from build123d import *

# Parameters (mm, degrees)
FILLET1_R = 2.54


with BuildPart() as part:
    # Sketch1 → Revolve2 (revolve)
    with BuildSketch(Plane.XY):
        Polygon((0, -25.4), (0, 25.4), (6.35, 25.4), (6.35, 3.175), (38.1, 3.175), (43.827481803, 18.715945904), (53.987481803, 18.715945904), (53.987481803, -18.715945904), (43.149559422, -18.715945904), (38.1, -3.175), (6.35, -3.175), (6.35, -25.4), align=None)
    revolve(axis=Axis((63.5, 0, 0), (0, 1, 0)))

    # Fillet1
    fillet1_edges = [part.edges().sort_by_distance(p)[0] for p in [
        (120.65, 25.4, 0),
        (127, 25.4, 0),
        (127, -25.4, 0),
    ]]
    fillet(fillet1_edges, radius=FILLET1_R)


solid = part.part
Could you check a few things on this model? Use its own coordinates, in mm. A direction names the side the tool comes from. Give positions to 0.01 mm unless a question says otherwise; leave off trailing zeros. Order: outer loops, then holes, each group sorted by start corner. A loop starts at its lowest first (then second) coordinate and runs counter-clockwise, first axis right, second up. Notation, with made-up numbers: (-14.5, 1.25) - (40.5, 1.25) arc R20 ccw to (40.5, 22.25) - close; hole circle Ø2 at (-36, 40.25). An arc over 180 degrees is marked (long way). One line per item, written item: value. Start each with the question number.
1. Thinking about a two-plate mould opening in Z: for faces 1 (the face through (75, -3.175, -25)), 2 (the face through (4.84, 0.32, -24.32)), 3 (the face through (81.3, -25.4, 54.5)), 4 (the face through (9, 12.9, 17.2)), which applies, +Z half, -Z half, draft (parallel to the pull), parting line (faces both ways), or undercut?
2. For faces 5 (the face through (68, -18.716, -9)), 6 (the face through (52, 3.175, -25)), 7 (the face through (54.427, -0.262, 2.857)), which set-ups out of +Z, -Z, +X, -X, +Y, -Y let a thin tool reach every point of the face, with its end or its side?
3. If I drill on probe 1 along X at (y, z) = (-12, -6.5); probe 2 along Z at (x, y) = (80, -4); probe 3 along X at (y, z) = (-14, -10), over which ranges is the centre line in solid material (lowest first)?
4. For P1, Ø10, axis at y = -1.5, z = -47.5, coming from the +X side; P2, Ø12, axis at x = 100.5, z = -34.5, coming from the -Y side (3 decimals); P3, Ø20.5, axis at x = 65.5, z = 4, coming from the -Y side, each with a flat end and sliding along its axis, tell me the tip position at first contact or that it passes through.
5. Imagine slicing it at C-C on y = 16. List the corners of the cut face in (x, z) for me, plus the area to 3 significant figures.
6. Imagine slicing it at D-D on y = -1. List the corners of the cut face in (x, z) for me.
Values:
1. face 1: undercut
1. face 2: parting line
1. face 3: draft
1. face 4: undercut
2. face 5: -Y
2. face 6: +Y
2. face 7: +Y, -Y
3. probe 1: 0.33 to 6.72, 41.93 to 56.55, 70.45 to 85.07, 120.28 to 126.67
3. probe 2: -61.32 to -54.72, -18.96 to 18.96, 54.72 to 61.32
3. probe 3: 0.79 to 7.23, 44.04 to 82.96, 119.77 to 126.21
4. P1: x = 110.68
4. P2: y = -3.175
4. P3: y = -18.72
5. outline: circle Ø127 at (63.5, 0); circle Ø41.35 at (63.5, 0); hole circle Ø114.3 at (63.5, 0); hole circle Ø19.03 at (63.5, 0)
5. area: 3,470 mm²
6. outline: circle Ø127 at (63.5, 0); hole circle Ø19.03 at (63.5, 0)
